```python
from build123d import *

# Parameters (mm, degrees)
BOSS_EXTRU_1_DEPTH           = 12
COQUE1_T                     = -2.6
ESQUISSE4_R                  = 7.5
BOSS_EXTRU_2_DEPTH           = 12.4
NERVURE1_REACH               = 28.407
ESQUISSE6_WALLS_W            = 1.5
ESQUISSE6_WALLS_H            = 61.384627196
R_P_TITION_CIRCULAIRE1_COUNT = 5
ESQUISSE7_R                  = 6
ENL_V_MAT_EXTRU_1_DEPTH      = 4.5
ENL_V_MAT_EXTRU_2_DEPTH      = 5


with BuildPart() as part:
    # Esquisse1 → Boss.-Extru.1 (new body)
    with BuildSketch(Plane.XY):
        with BuildLine():
            ThreePointArc((-6.475738253, 15.718295521), (-9.992349289, 13.753288904), (-12.947874208, 11.016013502))
            ThreePointArc((-12.947874208, 11.016013502), (-12.861203675, 4.178858391), (-16.950100551, -1.301572625))
            ThreePointArc((-16.950100551, -1.301572625), (-16.167960777, -5.253288904), (-14.477964596, -8.910024756))
            ThreePointArc((-14.477964596, -8.910024756), (-7.948661008, -10.940393303), (-4, -16.522711642))
            ThreePointArc((-4, -16.522711642), (0, -17), (4, -16.522711642))
            ThreePointArc((4, -16.522711642), (7.948661008, -10.940393303), (14.477964596, -8.910024756))
            ThreePointArc((14.477964596, -8.910024756), (16.167960777, -5.253288904), (16.950100551, -1.301572625))
            ThreePointArc((16.950100551, -1.301572625), (12.861203675, 4.178858391), (12.947874208, 11.016013502))
            ThreePointArc((12.947874208, 11.016013502), (9.992349289, 13.753288904), (6.475738253, 15.718295521))
            ThreePointArc((6.475738253, 15.718295521), (0, 13.523069823), (-6.475738253, 15.718295521))
        make_face()
    extrude(amount=BOSS_EXTRU_1_DEPTH)

    # Coque1
    coque1_openings = [part.faces().sort_by_distance(p)[0] for p in [
        (0, 0, 12),
    ]]
    offset(amount=COQUE1_T, openings=coque1_openings, kind=Kind.INTERSECTION)

    # Esquisse4 → Boss.-Extru.2 (add)
    with BuildSketch(Plane.XY.offset(15)):
        Circle(ESQUISSE4_R)
    extrude(amount=-BOSS_EXTRU_2_DEPTH)

    # Esquisse6 walls → Nervure1 (add, up to next)
    with BuildSketch(Plane.XY.offset(11), mode=Mode.PRIVATE) as nervure1_sk1:
        with Locations((0, 9.152971246)):
            Rectangle(ESQUISSE6_WALLS_W, ESQUISSE6_WALLS_H)
    nervure1_tool1 = extrude(nervure1_sk1.sketch, amount=-NERVURE1_REACH, mode=Mode.PRIVATE) - part.part
    nervure1 = nervure1_tool1.solids().sort_by_distance((0, 9.152971246, 11))[0]
    add(nervure1)

    # Répétition circulaire1: Nervure1 ×5 about axis
    r_p_tition_circulaire1_axis = Axis((0, 0, 0), (0, 0, 1))
    for i in range(1, R_P_TITION_CIRCULAIRE1_COUNT):
        add(nervure1.rotate(r_p_tition_circulaire1_axis, i * 360 / R_P_TITION_CIRCULAIRE1_COUNT))

    # Esquisse7 → Enlèv. mat.-Extru.1 (cut)
    with BuildSketch(Plane(origin=(0, 0, 0), x_dir=(-1, 0, 0), z_dir=(0, 0, -1))):
        Circle(ESQUISSE7_R)
    extrude(amount=-ENL_V_MAT_EXTRU_1_DEPTH, mode=Mode.SUBTRACT)

    # Esquisse8 → Enlèv. mat.-Extru.2 (cut)
    with BuildSketch(Plane.XY.offset(15)):
        Polygon((-5, 2.886751346), (-5, -2.886751346), (0, -5.773502692), (5, -2.886751346), (5, 2.886751346), (0, 5.773502692), align=None)
    extrude(amount=-ENL_V_MAT_EXTRU_2_DEPTH, mode=Mode.SUBTRACT)


solid = part.part
```
Geometry: final body of the model. Coordinates: model frame, mm. A direction names the side the tool comes from. Coordinates: 2 decimals unless noted, no trailing zeros. Write each loop counter-clockwise with the first axis right and the second up, starting at its lowest first coordinate (ties: lowest second). Pieces come first, ordered by that corner, then holes. Notation, with made-up numbers: M 68.5,41 L 99.5,41 A24 cw 99.5,60 Z; hole C -4,27.5 d1. An arc over 180 degrees is marked long. Use CSV: the item, a comma, the result in double quotes. Start each with the question number.
1. Cut plane B-B on y = 14. Return the cut outline in (x, z).
2. Reachability of faces 1 (the face through (-12.83, 4.27, 5.92)), 2 (the face through (-13.704, -4.422, 7.234)), 3 (the face through (6, 0, 2)) from +Z, -Z, +X, -X, +Y, -Y: full face, straight path, thin tool, end or side. Return the list, or none.
3. Ray query, probe 1 along X at (y, z) = (7.5, 10.25); probe 2 along X at (y, z) = (4.5, 8); probe 3 along X at (y, z) = (11, 1.5). Return the intervals inside material, ascending.
4. First-contact query: P1, Ø7.5, axis at x = -4.5, y = 8.5, coming from the +Z side; P2, Ø3, axis at x = 2, y = 0.5, coming from the +Z side; P3, Ø4, axis at y = 5.5, z = 12, coming from the +X side; P4, Ø3.5, axis at x = 5.5, y = -7.5, coming from the +Z side. Flat tips, straight axial feed; report the tip coordinate or a pass-through.
5. Cut plane C-C on y = -10. Return the cut outline in (x, z), plus the area to 3 significant figures.
6. Cut plane A-A on z = 11.5. Return the cut outline in (x, y), plus the area to 3 significant figures.
7. Cut plane D-D on z = 9. Count the separate pieces of the cut face and the enclosed holes in it, plus the area to 3 significant figures.
8. Mould query, pull axis Y, two halves, no side actions, for faces 4 (the face through (-5.952, -4.564, 8.887)), 5 (the face through (-9.947, 13.786, 5.916)). Classes: pulls with the +Y half, pulls with the -Y half, needs draft (parallel to the pull), parting line crosses it, or undercut.
Entries:
1,outline,"M -9.64,0 L -3.15,0 L -3.15,12 L -9.64,12 Z; M 3.15,0 L 9.64,0 L 9.64,12 L 3.15,12 Z"
2,face 1,"+Z, -Z, -X"
2,face 2,"+Z"
2,face 3,"-Z"
3,probe 1,"-12.34 to -9.74, -0.75 to 0.75, 9.74 to 12.34"
3,probe 2,"-12.76 to -10.08, -6 to 6, 10.08 to 12.76"
3,probe 3,"-12.94 to 12.94"
4,P1,"z = 15"
4,P2,"z = 10"
4,P3,"x = 13.11"
4,P4,"z = 12"
5,outline,"M -9.51,0 L 9.51,0 L 9.51,12 L 5.03,12 L 5.03,2.6 L -5.03,2.6 L -5.03,12 L -9.51,12 Z"
5,area,"134 mm²"
6,outline,"M -16.95,-1.3 A17 ccw -14.48,-8.91 A10.65 cw -4,-16.52 A17 ccw 4,-16.52 A10.65 cw 14.48,-8.91 A17 ccw 16.95,-1.3 A10.65 cw 12.95,11.02 A17 ccw 6.48,15.72 A10.65 cw -6.48,15.72 A17 ccw -12.95,11.02 A10.65 cw Z; C 0,0 d15; hole M -14.19,-2.44 A14.4 ccw -12.91,-6.37 A13.25 cw -2.07,-14.25 A14.4 ccw 2.07,-14.25 A13.25 cw 12.91,-6.37 A14.4 ccw 14.19,-2.44 A13.25 cw 10.05,10.31 A14.4 ccw 6.7,12.74 A13.25 cw -6.7,12.74 A14.4 ccw -10.05,10.31 A13.25 cw Z; hole M -5,-2.89 L 0,-5.77 L 5,-2.89 L 5,2.89 L 0,5.77 L -5,2.89 Z"
6,area,"351 mm²"
7,separate pieces,"1"
7,enclosed holes,"5"
7,area,"464 mm²"
8,face 4,"undercut"
8,face 5,"pulls with the +Y half"
